from build123d import *

# Parameters (mm, degrees)
CUT_EXTRUDE1_START   = -0.299999985
CUT_EXTRUDE1_DEPTH   = 0.099999976
CUT_EXTRUDE1_2_DEPTH = 0.624999986
CUT_EXTRUDE2_REACH   = 3.369
CUT_EXTRUDE3_DEPTH   = 0.099999976
CUT_EXTRUDE4_DEPTH   = 2.439835087
SKETCH8_W            = 0.45707022
SKETCH8_H            = 0.126497466
CUT_EXTRUDE5_DEPTH   = 2.36862159
BOSS_EXTRUDE1_DEPTH  = 0.3
SKETCH10_W           = 0.320867719
SKETCH10_H           = 0.471779159
BOSS_EXTRUDE2_DEPTH  = 0.1
CUT_EXTRUDE6_DEPTH   = 2.347497156
SKETCH12_W           = 0.905202631
SKETCH12_H           = 0.17588134
CUT_EXTRUDE7_DEPTH   = 2.347497156
SKETCH13_W           = 2.413938714
SKETCH13_H           = 1.247285026
CUT_EXTRUDE8_DEPTH   = 0.03
SKETCH14_W           = 2.254507246
SKETCH14_H           = 1.130570224
CUT_EXTRUDE9_DEPTH   = 0.001
SCALE1_SCALE         = 26


with BuildPart() as part:
    # Cut-Extrude1: read off the stored shape, not the designer's step
    # Cut-Extrude1 outline → Cut-Extrude1 (new body)
    with BuildSketch(Plane(origin=(0, 0, 0), x_dir=(-1, 0, 0), z_dir=(0, 1, 0)).offset(CUT_EXTRUDE1_START)):
        Polygon((-0.103293976, 1.023100922), (-0.125000006, 1.025000005), (-0.500000024, 1.025000005), (-0.52170601, 1.023100922), (-0.542752503, 1.017461531), (-0.562499976, 1.008253195), (-0.580348424, 0.995755661), (-0.595755526, 0.980348443), (-0.608253176, 0.962500053), (-0.61746157, 0.942752522), (-0.623101019, 0.921706087), (-0.624999986, 0.899999985), (-0.624999986, -1.025000005), (-0.623101019, -1.046706107), (-0.61746157, -1.067752484), (-0.608253176, -1.087500015), (-0.595755526, -1.105348463), (-0.580348424, -1.120755565), (-0.562499976, -1.133253216), (-0.542752503, -1.142461551), (-0.52170601, -1.148100942), (-0.500000024, -1.150000026), (-0.125000006, -1.150000026), (-0.103293976, -1.148100942), (-0.082247483, -1.142461551), (-0.062500003, -1.133253216), (-0.044651548, -1.120755565), (-0.029244446, -1.105348463), (-0.016746824, -1.087500015), (-0.007538422, -1.067752484), (-0.001899031, -1.046706107), (0, -1.025000005), (0, 0.899999985), (-0.001899031, 0.921706087), (-0.007538422, 0.942752522), (-0.016746824, 0.962500053), (-0.029244446, 0.980348443), (-0.044651548, 0.995755661), (-0.062500003, 1.008253195), (-0.082247483, 1.017461531), align=None)
    extrude(amount=CUT_EXTRUDE1_DEPTH)

    # Cut-Extrude1 2 outline → Cut-Extrude1 2 (add)
    with BuildSketch(Plane.YZ):
        Polygon((0.057826259, 0.496644876), (0, 0.500000024), (-0.200000009, 0.500000024), (-0.200000009, -0.73204824), (-0.155237081, -0.710894703), (-0.114767128, -0.682375045), (-0.079790305, -0.647334848), (-0.051343839, -0.60681341), (-0.030271342, -0.562012312), (-0.023619925, -0.547616393), (-0.014776401, -0.534452964), (-0.003963165, -0.522853108), (0.008547848, -0.513108505), (0.022442007, -0.505464152), (0.037369897, -0.500112365), (0.0529561, -0.497187721), (0.110784524, -0.487572339), (0.167090067, -0.471254607), (0.22109873, -0.448458857), (0.272068108, -0.41949845), (0.319297513, -0.384771498), (0.362137827, -0.344755303), (0.400000019, -0.299999985), (0.400000019, 0.299999985), (0.362620107, 0.344247906), (0.320373714, 0.383875886), (0.273827725, 0.418351992), (0.223606796, 0.447213592), (0.170384956, 0.47007337), (0.114876457, 0.486624485), align=None)
    extrude(amount=CUT_EXTRUDE1_2_DEPTH)

    # Sketch2 → Cut-Extrude2 (cut, up to next)
    with BuildSketch(Plane.ZY, mode=Mode.PRIVATE) as cut_extrude2_sk1:
        Polygon((-0.65000006, -0.299999985), (0.400000019, -0.299999985), (0.400000019, 0), (0.396011048, 0.056349407), (0.384123705, 0.11157494), (0.364575157, 0.164575133), (0.337755162, 0.214292915), (0.304198737, 0.259736669), (0.264575152, 0.299999985), (-0.264575152, 0.299999985), (-0.299557927, 0.265075563), (-0.329965871, 0.226102915), (-0.355334574, 0.183677243), (-0.375276693, 0.138446456), (-0.389487541, 0.091101319), (-0.397750206, 0.042364885), (-0.403599464, 0.011192467), (-0.414303038, -0.01866331), (-0.429591688, -0.046451623), (-0.449080922, -0.07147366), (-0.472280721, -0.093100134), (-0.498607522, -0.110787172), (-0.527399301, -0.124090002), (-0.556858547, -0.137973097), (-0.583471148, -0.15674415), (-0.606434362, -0.179836949), (-0.625055342, -0.20655476), (-0.638772442, -0.236091611), (-0.647171808, -0.267556432), align=None)
    cut_extrude2_tool1 = extrude(cut_extrude2_sk1.sketch, amount=-CUT_EXTRUDE2_REACH, mode=Mode.PRIVATE) & part.part
    add(cut_extrude2_tool1.solids().sort_by_distance((0, -0.029264, -0.044377))[0], mode=Mode.SUBTRACT)

    # Sketch3 → Cut-Extrude3 (cut)
    with BuildSketch(Plane(origin=(0, -0.200000009, 0), x_dir=(-1, 0, 0), z_dir=(0, 1, 0))):
        Polygon((-0.231526632, 0.946749991), (-0.240874855, 0.960100675), (-0.252399361, 0.971625152), (-0.265749986, 0.98097336), (-0.280521112, 0.987861305), (-0.296263897, 0.992079498), (-0.312499993, 0.993499998), (-0.328736118, 0.992079498), (-0.344478874, 0.987861305), (-0.359249971, 0.98097336), (-0.372600654, 0.971625152), (-0.38412516, 0.960100675), (-0.393473398, 0.946749991), (-0.400361256, 0.931978866), (-0.404579536, 0.91623608), (-0.405999977, 0.899999985), (-0.405999977, 0.713000074), (-0.404579536, 0.69676392), (-0.400361256, 0.681021134), (-0.393473398, 0.666250009), (-0.38412516, 0.652899384), (-0.372600654, 0.641374907), (-0.359249971, 0.63202664), (-0.344478874, 0.625138753), (-0.328736118, 0.620920502), (-0.312499993, 0.619500061), (-0.296263897, 0.620920502), (-0.280521112, 0.625138753), (-0.265749986, 0.63202664), (-0.252399361, 0.641374907), (-0.240874855, 0.652899384), (-0.231526632, 0.666250009), (-0.224638745, 0.681021134), (-0.220420479, 0.69676392), (-0.219000009, 0.713000074), (-0.219000009, 0.899999985), (-0.220420479, 0.91623608), (-0.224638745, 0.931978866), align=None)
    extrude(amount=-CUT_EXTRUDE3_DEPTH, mode=Mode.SUBTRACT)

    # Sketch4 → Cut-Extrude4 (cut, through all)
    with BuildSketch(Plane(origin=(0, -0.200000009, 0), x_dir=(-1, 0, 0), z_dir=(0, 1, 0))):
        Polygon((-0.393473398, -1.07175007), (-0.38412516, -1.085100695), (-0.372600654, -1.09662523), (-0.359249971, -1.105973381), (-0.344478874, -1.112861326), (-0.328736118, -1.117079635), (-0.312499993, -1.118500018), (-0.296263897, -1.117079635), (-0.280521112, -1.112861326), (-0.265749986, -1.105973381), (-0.252399361, -1.09662523), (-0.240874855, -1.085100695), (-0.231526632, -1.07175007), (-0.224638745, -1.056978945), (-0.220420479, -1.041236101), (-0.219000009, -1.025000005), (-0.219000009, -0.837999978), (-0.220420479, -0.821763941), (-0.224638745, -0.806021097), (-0.231526632, -0.791249971), (-0.240874855, -0.777899404), (-0.252399361, -0.766374869), (-0.265749986, -0.757026661), (-0.280521112, -0.750138774), (-0.296263897, -0.745920464), (-0.312499993, -0.744499965), (-0.328736118, -0.745920464), (-0.344478874, -0.750138774), (-0.359249971, -0.757026661), (-0.372600654, -0.766374869), (-0.38412516, -0.777899404), (-0.393473398, -0.791249971), (-0.400361256, -0.806021097), (-0.404579536, -0.821763941), (-0.405999977, -0.837999978), (-0.405999977, -1.025000005), (-0.404579536, -1.041236101), (-0.400361256, -1.056978945), align=None)
    extrude(amount=-CUT_EXTRUDE4_DEPTH, mode=Mode.SUBTRACT)

    # Sketch8 → Cut-Extrude5 (cut, through all)
    with BuildSketch(Plane(origin=(0, 0, 0), x_dir=(0, 0, -1), z_dir=(1, 0, 0))):
        with Locations((0.96058335, -0.263248742)):
            Rectangle(SKETCH8_W, SKETCH8_H)
    extrude(amount=CUT_EXTRUDE5_DEPTH, mode=Mode.SUBTRACT)

    # Sketch9 → Boss-Extrude1 (add)
    with BuildSketch(Plane(origin=(0, 0, -0.73204824), x_dir=(-1, 0, 0), z_dir=(0, 0, -1))):
        Polygon((0, -0.299999985), (0, -0.200000009), (-0.624999986, -0.200000009), (-0.624999986, -0.278120473), (-0.624999986, -0.299999985), (-0.529422539, -0.299999985), (-0.519709533, -0.299999985), (-0.506867205, -0.299999985), (-0.490512573, -0.299999985), (-0.470477371, -0.299999985), (-0.447049913, -0.299999985), (-0.421272081, -0.299999985), (-0.395156344, -0.299999985), (-0.371582464, -0.299999985), (-0.353676372, -0.299999985), (-0.271323614, -0.299999985), (-0.253417547, -0.299999985), (-0.229843642, -0.299999985), (-0.203727882, -0.299999985), (-0.177950094, -0.299999985), (-0.154522634, -0.299999985), (-0.134487439, -0.299999985), (-0.118132789, -0.299999985), (-0.105290467, -0.299999985), (-0.095577447, -0.299999985), (-0.047916146, -0.299999985), align=None)
    extrude(amount=BOSS_EXTRUDE1_DEPTH)

    # Sketch10 → Boss-Extrude2 (add, through all)
    with BuildSketch(Plane(origin=(0, -0.200000009, 0), x_dir=(-1, 0, 0), z_dir=(0, 1, 0))):
        with Locations((-0.31112302, 0.768217279)):
            Rectangle(SKETCH10_W, SKETCH10_H)
    extrude(amount=-BOSS_EXTRUDE2_DEPTH)

    # Sketch11 → Cut-Extrude6 (cut, through all)
    with BuildSketch(Plane(origin=(0, -0.200000009, 0), x_dir=(-1, 0, 0), z_dir=(0, 1, 0))):
        with BuildLine():
            Line((-0.381567202, 0.602069646), (-0.381567202, 0.742122646))
            ThreePointArc((-0.381567202, 0.742122646), (-0.321550512, 0.802139336), (-0.261533822, 0.742122646))
            Line((-0.261533822, 0.742122646), (-0.261533822, 0.602069646))
            ThreePointArc((-0.261533822, 0.602069646), (-0.321550512, 0.542052956), (-0.381567202, 0.602069646))
        make_face()
    extrude(amount=-CUT_EXTRUDE6_DEPTH, mode=Mode.SUBTRACT)

    # Sketch12 → Cut-Extrude7 (cut, through all)
    with BuildSketch(Plane(origin=(0, -0.200000009, 0), x_dir=(-1, 0, 0), z_dir=(0, 1, 0))):
        with Locations((-0.289049147, 0.960305627)):
            Rectangle(SKETCH12_W, SKETCH12_H)
    extrude(amount=-CUT_EXTRUDE7_DEPTH, mode=Mode.SUBTRACT)

    # Sketch13 → Cut-Extrude8 (cut)
    with BuildSketch(Plane(origin=(0.624999986, 0, 0), x_dir=(0, 0, -1), z_dir=(1, 0, 0))):
        Rectangle(SKETCH13_W, SKETCH13_H)
    extrude(amount=-CUT_EXTRUDE8_DEPTH, mode=Mode.SUBTRACT)

    # Sketch14 → Cut-Extrude9 (cut)
    with BuildSketch(Plane.ZY):
        Rectangle(SKETCH14_W, SKETCH14_H)
    extrude(amount=-CUT_EXTRUDE9_DEPTH, mode=Mode.SUBTRACT)


with BuildPart() as part_1:
    # Scale1: scaled about (0.297584829, 0.035955959, -0.052860466)
    add(part.part.scale(SCALE1_SCALE).moved(Location((-7.439620725, -0.898898975, 1.32151165))))


solid = part_1.part
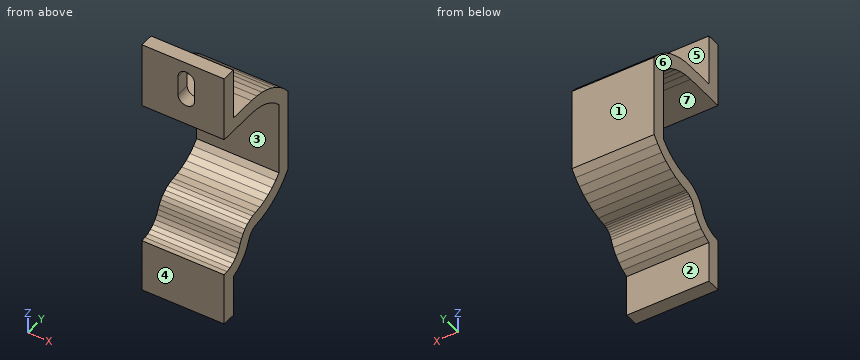
The listing builds one solid part. Answer for the finished solid, in the listing's coordinates (mm). Face numbers are marked on the shaded views. A direction names the side the tool comes from. Round coordinates to 2 decimals unless told otherwise and drop trailing zeros. Write each loop counter-clockwise with the first axis right and the second up, starting at its lowest first coordinate (ties: lowest second). Pieces come first, ordered by that corner, then holes. Notation, with made-up numbers: (-38.75, 2.25) - (12.25, 2.25) arc R13 ccw to (12.25, 21.25) - close; hole circle Ø3 at (48.25, -35.5). An arc over 180 degrees is marked (long way). Use one line per item in the form item = value. Start each with the question number.
Item 1: Flat-ended cylindrical pins translate along their axes: pin 1 Ø4 at (x, y) = (2.5, -4.5) entering from +Z; pin 2 Ø1 at (x, y) = (0, -1.5) entering from +Z; pin 3 Ø1.5 at (x, y) = (0, 1.5) entering from -Z; pin 4 Ø8.5 at (x, z) = (3.5, -22) entering from +Y. Find the tip coordinate at first contact, or state that the pin passes through.
Item 2: A cutting plane is placed at A-A (z = 19). Write down the section's boundary in (x, y), plus the area to 3 significant figures.
Item 3: Determine the mould class of the marked faces 6 and 7 for opening direction Z: +Z half, -Z half, draft (parallel to the pull), parting line (faces both ways), or undercut.
Item 4: A cutting plane is placed at B-B (z = 2). Write down the section's boundary in (x, y).
Item 5: Find the intervals of material crossed by line 1 (Y direction, x = 0.25, z = -1.5); line 2 (Y direction, x = 2.5, z = 16); line 3 (Z direction, x = 3, y = 2.25), in increasing order. Write a range as [from, to].
Item 6: A tool of negligible diameter and unlimited length cuts with its end or side. For the marked faces 1, 2, 3, 4 and 5, from which of +Z, -Z, +X, -X, +Y, -Y can it reach the whole face along a straight path? Write none if from no direction.
The answers:
q1.pin_1 = 24
q1.pin_2 = 14.32
q1.pin_3 = -11.56
q1.pin_4 = -6.1
q2.outline = (-7.41, -8.7) - (-0.64, -8.7) - (-0.64, -6.1) - (-7.41, -6.1) - close; (2.48, -8.7) - (8.03, -8.7) - (8.03, -6.1) - (2.48, -6.1) - close
q2.area = 32.0 mm^2
q3.face_6 = draft
q3.face_7 = undercut
q4.outline = (-7.41, 6.9) - (8.03, 6.9) - (8.03, 9.5) - (-7.41, 9.5) - close
q5.line_1 = [6.9, 9.5]
q5.line_2 = [-8.7, -6.1]
q5.line_3 = [-11.28, -8.57], [11.22, 13.93]
q6.face_1 = +Z, -Z, +X, -X, +Y
q6.face_2 = -Z, +X, -X, +Y
q6.face_3 = +X, -X, -Y
q6.face_4 = +Z, -Z, +X, -X, -Y
q6.face_5 = +Z, +X, -X, +Y
